```python
from build123d import *

# Parameters (mm, degrees)
SKETCH3_W          = 1.016
SKETCH3_H          = 1.016
CHAMFER1_SIZE      = 0.5159375
SKETCH2_R          = 0.762
CUT_EXTRUDE1_DEPTH = 2.54
CHAMFER2_SIZE      = 0.254
CHAMFER2_SIZE_2    = 0.209783356


with BuildPart() as part:
    # Sketch1 → Revolve1 (revolve)
    with BuildSketch(Plane(origin=(0, 0, 0), x_dir=(0, 0, -1), z_dir=(1, 0, 0)), mode=Mode.PRIVATE) as revolve1_sk:
        with BuildLine():
            Line((0, 0), (0, 5.159375))
            Line((0, 5.159375), (-9.525, 5.159375))
            Line((-9.525, 5.159375), (-9.525, 7.14375))
            Line((-9.525, 7.14375), (-11.10615, 7.14375))
            Line((-11.10615, 7.14375), (-11.10615, 3.175))
            Line((-11.10615, 3.175), (-13.586546081, 3.175))
            ThreePointArc((-13.586546081, 3.175), (-15.831610111, 2.24506403), (-16.761546081, 0))
            Line((-16.761546081, 0), (0, 0))
        make_face()
    revolve(revolve1_sk.sketch.rotate(Axis((0, 0, 17.430941175), (0, 0, -1)), 90), axis=Axis((0, 0, 17.430941175), (0, 0, -1)))

    # Sketch3 → Cut-Revolve1 (revolve, cut)
    with BuildSketch(Plane(origin=(0, 0, 0), x_dir=(0, 0, -1), z_dir=(1, 0, 0)), mode=Mode.PRIVATE) as cut_revolve1_sk:
        with Locations((-11.36015, 3.429)):
            Rectangle(SKETCH3_W, SKETCH3_H)
        with Locations((-9.271, 5.413375)):
            Rectangle(SKETCH3_W, SKETCH3_H)
    revolve(cut_revolve1_sk.sketch.rotate(Axis((0, 0, 17.430941175), (0, 0, -1)), 90), axis=Axis((0, 0, 17.430941175), (0, 0, -1)), mode=Mode.SUBTRACT)

    # Chamfer1
    chamfer1_edges = [part.edges().sort_by_distance(p)[0] for p in [
        (-5.159375, 0, 0),
    ]]
    chamfer(chamfer1_edges, length=CHAMFER1_SIZE)

    # Sketch2 → Cut-Extrude1 (cut)
    with BuildSketch(Plane(origin=(0, 0, 0), x_dir=(-1, 0, 0), z_dir=(0, 0, -1))):
        Circle(SKETCH2_R)
    cut_extrude1 = extrude(amount=-CUT_EXTRUDE1_DEPTH, mode=Mode.SUBTRACT)

    # Mirror1: Cut-Extrude1 across plane
    add(cut_extrude1.mirror(Plane.XY.offset(8.38077304)), mode=Mode.SUBTRACT)

    # Chamfer2
    # the kernel refuses this chamfer: 0.254, 0.209783356 mm, written as the material it takes off along each edge
    with BuildSketch(Plane(origin=(0, 0, 0), x_dir=(-1, 0, 0), z_dir=(0, -1, 0))) as chamfer2_piece_1:
        Polygon((0.762 + CHAMFER2_SIZE, 0), (0.762, -CHAMFER2_SIZE), (0.762, 0), align=None)
    revolve(axis=Axis((0, 0, 0), (0, 0, -1)), mode=Mode.SUBTRACT)
    with BuildSketch(Plane(origin=(0, 0, 16.66875), x_dir=(-1, 0, 0), z_dir=(0, 1, 0))) as chamfer2_piece_2:
        with BuildLine():
            Line((0.997154658, -0.067853643), (0.762, -CHAMFER2_SIZE_2))
            Line((0.762, -CHAMFER2_SIZE_2), (0.762, 0))
            ThreePointArc((0.762, 0), (0.883545152, -0.032618216), (0.997154658, -0.067853643))
        make_face()
    revolve(axis=Axis((0, 0, 16.66875), (0, 0, 1)), revolution_arc=180, mode=Mode.SUBTRACT)
    with BuildSketch(Plane(origin=(0, 0, 16.66875), x_dir=(1, 0, 0), z_dir=(0, -1, 0))) as chamfer2_piece_3:
        with BuildLine():
            Line((0.997154658, -0.067853643), (0.762, -CHAMFER2_SIZE_2))
            Line((0.762, -CHAMFER2_SIZE_2), (0.762, 0))
            ThreePointArc((0.762, 0), (0.883545152, -0.032618216), (0.997154658, -0.067853643))
        make_face()
    revolve(axis=Axis((0, 0, 16.66875), (0, 0, 1)), revolution_arc=180, mode=Mode.SUBTRACT)


solid = part.part
```
Can you work these out from the model? Positions are in its coordinate system, mm. A direction names the side the tool comes from. Give positions to 0.01 mm unless a question says otherwise; leave off trailing zeros. Write each loop counter-clockwise with the first axis right and the second up, starting at its lowest first coordinate (ties: lowest second). Pieces come first, ordered by that corner, then holes. Notation, with made-up numbers: (69.25, 54) -> (110.25, 54) arc R35 cw to (110.25, 91) -> close; hole circle Ø11 at (-24.75, 25.5). An arc over 180 degrees is marked (long way). Write item = value, one per line.
(1) I'm going to push flat-ended pins straight in: P1, Ø5, axis at x = -1.5, y = 1.5, coming from the +Z side; P2, Ø0.9, axis at x = 0, y = 0, coming from the +Z side; P3, Ø4, axis at y = -5, z = 5, coming from the -X side; P4, Ø1.9, axis at x = 0, y = 0, coming from the -Z side. Where does each tip first touch, or does it pass through?
Worked out:
P1 = 16.6
P2 = 14.22
P3 = -4.2
P4 = 0.07
(2) I need wall thicknesses on probe 1 along Y at (x, z) = (0, 11); probe 2 along Y at (x, z) = (0, 2.15); probe 3 along Z at (x, y) = (3.75, -3.75). Which ranges of each line are inside material? Lowest first, please. Write a range as from..to.
Worked out:
probe_1 = -7.14..-3.94, -2.92..2.92, 3.94..7.14
probe_2 = -5.16..-0.76, 0.76..5.16
probe_3 = 9.78..11.11
(3) Suppose I cut it at B-B on y = 5.5. Write out the boundary of the cut face in (x, z) (3 decimals).
Worked out:
outline = (-4.559, 9.525) -> (-2.194, 9.525) -> (-2.194, 9.779) -> (2.194, 9.779) -> (2.194, 9.525) -> (4.559, 9.525) -> (4.559, 11.106) -> (-4.559, 11.106) -> close
(4) Suppose I cut it at D-D on z = 4.5. Write out the boundary of the cut face in (x, y).
Worked out:
outline = circle Ø10.32 at (0, 0)
(5) Thinking about a two-plate mould opening in Y: for faces 1 (the face through (3, 3, 11.106)), 2 (the face through (0, 0, 2.54)), 3 (the face through (-7.137, -0.314, 10.327)), which applies, released by +Y, released by -Y, zero draft, split by the parting line, or undercut?
Worked out:
face_1 = zero draft
face_2 = undercut
face_3 = split by the parting line
(6) Suppose I cut it at C-C on z = 14.5. Write out the boundary of the cut face in (x, y), then the cut area to 3 significant figures.
Worked out:
outline = circle Ø6.08 at (0, 0); hole circle Ø1.52 at (0, 0)
area = 27.2 mm^2
(7) Suppose I cut it at A-A on z = 10.25. Write out the boundary of the cut face in (x, y), then the cut area to 3 significant figures.
Worked out:
outline = circle Ø14.29 at (0, 0)
area = 160 mm^2
(8) For faces 4 (the face through (-1, -6, 9.525)), 5 (the face through (0, 0, 14.222)), 6 (the face through (2.637, -4.136, 9.264)), 7 (the face through (-1, 1, 0)), which set-ups out of +Z, -Z, +X, -X, +Y, -Y let a thin tool reach every point of the face, with its end or its side?
Worked out:
face_4 = -Z
face_5 = +Z
face_6 = none
face_7 = -Z, +X, -X, +Y, -Y
